Read the model definition and answer for the solid it produces. Units are mm, in the model's axes. A direction names the side the tool comes from. Give positions to 0.01 mm unless a question says otherwise; leave off trailing zeros. Order: outer loops, then holes, each group sorted by start corner. A loop starts at its lowest first (then second) coordinate and runs counter-clockwise, first axis right, second up.
Item 1: Which of the six approach directions +Z, -Z, +X, -X, +Y, -Y give full straight-line access (tool end or side, diameter ignored) to faces 1 (the face through (-45.207, 3.5, -13.916)), 2 (the face through (0, -4, 0)), 3 (the face through (-35, -4, 1.3))?
Item 2: A cutting plane is placed at B-B (y = 36). State how many separate pieces and enclosed holes the cut face has, plus the area to 3 significant figures.
Item 3: Given pin 1 Ø10 at (x, y) = (-10, 1) entering from -Z; pin 2 Ø19 at (x, y) = (2.5, -111.5) entering from +Z; pin 3 Ø11 at (x, y) = (-40.5, -111) entering from -Z, each flat-ended and moving along its own axis, determine where each tip first touches the part or whether it passes through.
Item 4: Find the intervals of material crossed by line 1 along X through (y, z) = (125, -6.5); line 2 along X through (y, z) = (52, -7); line 3 along X through (y, z) = (-110, -16.25), in increasing order.
Item 5: A cutting plane is placed at C-C (x = 12). Write down the section's boundary in (y, z), plus the area to 3 significant figures.
Item 6: A cutting plane is placed at A-A (x = -7). Write down the section's boundary in (y, z).
Item 7: The mould has two halves that part along X. Classify faces 4 (the face through (-47.03, -3.5, -15.172)), 5 (the face through (36, -4, 1.3)), 6 (the face through (21, -4, -10)): +X half, -X half, draft (parallel to the pull), parting line (faces both ways), or undercut.
from build123d import *

# Parameters (mm, degrees)
F1_DEPTH    = 250
F2_W        = 38
F2_H        = 13
F3_DEPTH    = 250
F4_T1_DEPTH = 509.3674969976
F5_R        = 9
F6_R        = 1
F8_DEPTH    = 250


# Not quite as in the source:
# - a fillet or chamfer that OpenCascade refuses, or shapes differently, is made with other operations: its cross-section is extruded or revolved along the edge and cut away or added


with BuildPart() as f1:
    # F0 (on Front) → F1 (new body, symmetric)
    with BuildSketch(Plane.XZ):
        with BuildLine():
            Line((22.5, 0), (0, 0))
            Line((0, 0), (-22.5, 0))
            Line((-22.5, 0), (-22.5, 1.3))
            Line((-22.5, 1.3), (-49.8395555688, 1.3))
            Line((-49.8395555688, 1.3), (-57.5, -5.1278760969))
            Line((-57.5, -5.1278760969), (-57.5, -9.1278760969))
            Line((-57.5, -9.1278760969), (-33.9923918332, -22.7))
            ThreePointArc((-33.9923918332, -22.7), (0, -19.7901248096), (33.9923918332, -22.7))
            Line((33.9923918332, -22.7), (57.5, -9.1278760969))
            Line((57.5, -9.1278760969), (57.5, -5.1278760969))
            Line((57.5, -5.1278760969), (49.8395555688, 1.3))
            Line((49.8395555688, 1.3), (22.5, 1.3))
            Line((22.5, 1.3), (22.5, 0))
        make_face()
    extrude(amount=F1_DEPTH, both=True)

    # F2 (on Front) → F3 (cut, symmetric)
    with BuildSketch(Plane.XZ):
        with Locations((0, -8.5)):
            Rectangle(F2_W, F2_H)
    extrude(amount=F3_DEPTH, both=True, mode=Mode.SUBTRACT)

    # F4: fillet of radius 2 on 2 edges, made by hand

    # F4_s2 → F4_t1 (cut)
    with BuildSketch(Plane.XZ.offset(-254.6837484988)):
        with BuildLine():
            ThreePointArc((-24.3734993995, 1.3), (-23.2333239744, 0.9431676725), (-22.5, 0))
            Line((-22.5, 0), (-22.5, 1.3))
            Line((-22.5, 1.3), (-24.3734993995, 1.3))
        make_face()
        with BuildLine():
            ThreePointArc((24.3734993995, 1.3), (23.2333239744, 0.9431676725), (22.5, 0))
            Line((22.5, 0), (22.5, 1.3))
            Line((22.5, 1.3), (24.3734993995, 1.3))
        make_face()
    extrude(amount=F4_T1_DEPTH, mode=Mode.SUBTRACT)

    # F5
    f5_edges = [f1.edges().sort_by_distance(p)[0] for p in [
        (-49.839556, 0, 1.3),
        (49.839556, 0, 1.3),
        (33.992392, 0, -22.7),
        (-33.992392, 0, -22.7),
    ]]
    fillet(f5_edges, radius=F5_R)

    # F6
    f6_edges = [f1.edges().sort_by_distance(p)[0] for p in [
        (-57.5, 0, -5.127876),
        (57.5, 0, -5.127876),
        (57.5, 0, -9.127876),
        (-57.5, 0, -9.127876),
    ]]
    fillet(f6_edges, radius=F6_R)

    # F7 (on Front) → F8 (cut, symmetric)
    with BuildSketch(Plane.XZ):
        with BuildLine():
            ThreePointArc((-35.7777574473, -19.3598176053), (-33.5603570371, -20.1791322254), (-31.1966842313, -20.2136560239))
            ThreePointArc((-31.1966842313, -20.2136560239), (-26.106800057, -19.4842711987), (-21, -18.8846744107))
            Line((-21, -18.8846744107), (-21, -2))
            Line((-21, -2), (-22.5, -2))
            ThreePointArc((-22.5, -2), (-23.2333239744, -1.0568323275), (-24.3734993995, -0.7))
            Line((-24.3734993995, -0.7), (-46.5638234604, -0.7))
            ThreePointArc((-46.5638234604, -0.7), (-48.9579644637, -1.1221516545), (-51.0633367282, -2.3376888982))
            Line((-51.0633367282, -2.3376888982), (-54.6622869129, -5.3575666708))
            ThreePointArc((-54.6622869129, -5.3575666708), (-55.3691010897, -7.0639670425), (-54.3767116936, -8.6217063646))
            Line((-54.3767116936, -8.6217063646), (-35.7777574473, -19.3598176053))
        make_face()
        with BuildLine():
            Line((22.5, -2), (21, -2))
            Line((21, -2), (21, -18.8846744107))
            ThreePointArc((21, -18.8846744107), (26.106800057, -19.4842711987), (31.1966842313, -20.2136560239))
            ThreePointArc((31.1966842313, -20.2136560239), (33.5603570371, -20.1791322254), (35.7777574473, -19.3598176053))
            Line((35.7777574473, -19.3598176053), (54.3767116936, -8.6217063646))
            ThreePointArc((54.3767116936, -8.6217063646), (55.3691010897, -7.0639670425), (54.6622869129, -5.3575666708))
            Line((54.6622869129, -5.3575666708), (51.0633367282, -2.3376888982))
            ThreePointArc((51.0633367282, -2.3376888982), (48.9579644637, -1.1221516545), (46.5638234604, -0.7))
            Line((46.5638234604, -0.7), (24.3734993995, -0.7))
            ThreePointArc((24.3734993995, -0.7), (23.2333239744, -1.0568323275), (22.5, -2))
        make_face()
    extrude(amount=F8_DEPTH, both=True, mode=Mode.SUBTRACT)


solid = f1.part
Response values:
1. face 1: +Y, -Y
1. face 2: +Z, +Y, -Y
1. face 3: +Z, +X, -X, +Y, -Y
2. separate pieces: 1
2. enclosed holes: 3
2. area: 671 mm2
3. pin 1: stops at z = -20.35
3. pin 2: stops at z = 0
3. pin 3: stops at z = -21.88
4. line 1: x = -57.5 to -55.34, -21 to -19, 19 to 21, 55.34 to 57.5
4. line 2: x = -57.5 to -55.37, -21 to -19, 19 to 21, 55.37 to 57.5
4. line 3: x = -45.16 to -41.16, -21 to 21, 41.16 to 45.16
5. outline: (-250, -20.15) - (250, -20.15) - (250, -15) - (-250, -15) - close; (-250, -2) - (250, -2) - (250, 0) - (-250, 0) - close
5. area: 3,580 mm2
6. outline: (-250, -19.91) - (250, -19.91) - (250, -15) - (-250, -15) - close; (-250, -2) - (250, -2) - (250, 0) - (-250, 0) - close
7. face 4: -X half
7. face 5: draft
7. face 6: undercut
